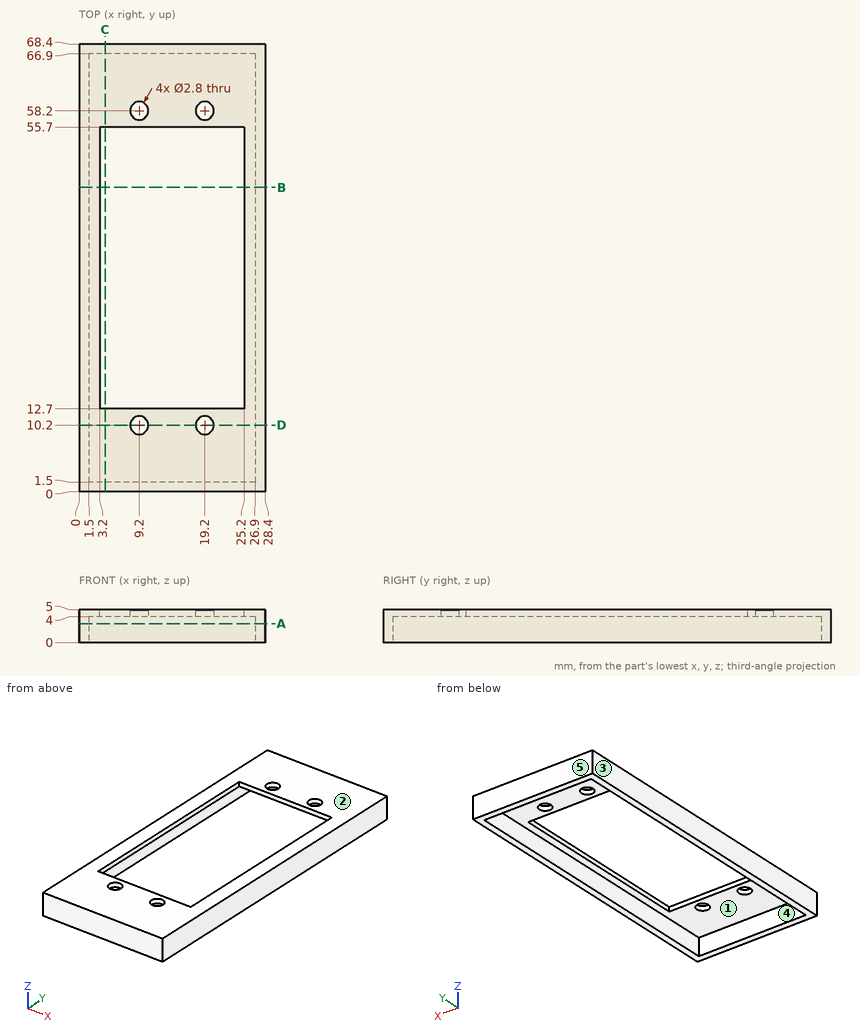
Job drawing, mm, ordinate dimensions from the low corner. One solid piece. A direction names the side the tool comes from. Coordinates: 2 decimals unless noted, no trailing zeros. Order: outer loops, then holes, each group sorted by start corner. A loop starts at its lowest first (then second) coordinate and runs counter-clockwise, first axis right, second up. Notation, with made-up numbers: (-12.75, 51.25) - (-4.75, 51.25) arc R21 cw to (-4.75, 62.25) - close; hole circle Ø9 at (41.25, 63.25). An arc over 180 degrees is marked (long way). Return JSON: item names as keys, results as strings. Group by question number.
1) Saw through at A-A, the plane z = 2.9. Write the cut outline in (x, y), plus the area to 3 significant figures.
2) Saw through at D-D, the plane y = 10.2. Write the cut outline in (x, z), plus the area to 3 significant figures.
3) Tool access for the marked faces 1 and 2: list every direction of +Z, -Z, +X, -X, +Y, -Y with a clear straight run to the whole face (end or side of a thin tool).
4) Saw through at C-C, the plane x = 4. Write the cut outline in (y, z), plus the area to 3 significant figures.
5) Saw through at B-B, the plane y = 46.5. Write the cut outline in (x, z), plus the area to 3 significant figures.
6) Probe line 1 (X direction, y = 58.2, z = 4.6); line 2 (Y direction, x = 19.2, z = 4.3); line 3 (X direction, y = 8, z = 2.5). List the from-to ranges inside material, lowest first. Write a range as from..to.
7) Flat gauge pins, fed straight in: P1, Ø4.5, axis at x = 19.2, y = 58.2, coming from the -Z side; P2, Ø6, axis at x = 23, y = 13.5, coming from the +Z side. Where does each tip first touch, or does it go through?
8) Mould opens along X. For the marked faces 3, 4 and 5 say: released by +X, released by -X, zero draft, split by the parting line, or undercut.
Values found:
{
 "1": {"outline": "(0, 0) - (28.4, 0) - (28.4, 68.4) - (0, 68.4) - close; hole (1.5, 1.5) - (26.9, 1.5) - (26.9, 66.9) - (1.5, 66.9) - close", "area": "281 mm²"},
 "2": {"outline": "(0, 0) - (1.5, 0) - (1.5, 4) - (7.8, 4) - (7.8, 5) - (0, 5) - close; (10.6, 4) - (17.8, 4) - (17.8, 5) - (10.6, 5) - close; (20.6, 4) - (26.9, 4) - (26.9, 0) - (28.4, 0) - (28.4, 5) - (20.6, 5) - close", "area": "34.8 mm²"},
 "3": {"face 1": "-Z", "face 2": "+Z, +X, -X, +Y, -Y"},
 "4": {"outline": "(0, 0) - (1.5, 0) - (1.5, 4) - (12.7, 4) - (12.7, 5) - (0, 5) - close; (55.7, 4) - (66.9, 4) - (66.9, 0) - (68.4, 0) - (68.4, 5) - (55.7, 5) - close", "area": "37.4 mm²"},
 "5": {"outline": "(0, 0) - (1.5, 0) - (1.5, 4) - (3.2, 4) - (3.2, 5) - (0, 5) - close; (25.2, 4) - (26.9, 4) - (26.9, 0) - (28.4, 0) - (28.4, 5) - (25.2, 5) - close", "area": "18.4 mm²"},
 "6": {"line 1": "x = 0..7.8, 10.6..17.8, 20.6..28.4", "line 2": "y = 0..8.8, 11.6..12.7, 55.7..56.8, 59.6..68.4", "line 3": "x = 0..1.5, 26.9..28.4"},
 "7": {"P1": "stops at z = 4", "P2": "stops at z = 5"},
 "8": {"face 3": "released by -X", "face 4": "undercut", "face 5": "zero draft"}
}
